Read the model definition and answer for the solid it produces. Units are mm, in the model's axes. Round coordinates to 2 decimals unless told otherwise and drop trailing zeros. Order: outer loops, then holes, each group sorted by start corner. A loop starts at its lowest first (then second) coordinate and runs counter-clockwise, first axis right, second up. Notation, with made-up numbers: M 30.25,73.5 L 40.25,73.5 A18 cw 40.25,94.5 Z; hole C 71,58.5 d10. An arc over 180 degrees is marked long. Use one line per item in the form item = value. Start each with the question number.
Autodesk Inventor part; units mm, degrees
ref_plane "Work Plane1" through (-6.3375, 0, 0) normal (0, -0.8660254, -0.5) x (1, 0, 0)
ref_plane "YZ Plane" through (0, 0, 0) normal (1, 0, 0) x (0, 1, 0)
ref_plane "XZ Plane" through (0, 0, 0) normal (0, 1, 0) x (-1, 0, 0)
sketch "Sketch1" plane through (0, 0, 0) normal (1, 0, 0) x (0, 1, 0)
  line L0 (-3.1754, 0) -> (-1.5877, 2.75)
  line L1 (-1.5877, 2.75) -> (1.5877, 2.75)
  line L2 (1.5877, 2.75) -> (3.1754, 0)
  line L3 (3.1754, 0) -> (1.5877, -2.75)
  line L4 (1.5877, -2.75) -> (-1.5877, -2.75)
  line L5 (-1.5877, -2.75) -> (-3.1754, 0)
  point P0 (0, 0)
  point P1 (0, 0)
  dimension "d0" = 6.3509
extrude "Body" add sketch "Sketch1" along normal blind 2.4
sketch "Sketch2" plane through (0, 0, 0) normal (0, 0, 1) x (1, 0, 0)
  line L0 (0, 1.5877) -> (0, 3.1754)
  line L1 (0, 3.1754) -> (2.4, 3.1754)
  line L2 (2.4, 1.5877) -> (2.4, 3.1754)
  line L3 (-0.16, 0) -> (0.96, 0)
  line L4 (0.1984, 3.1754) -> (0, 2.75)
  line L5 (2.2016, 3.1754) -> (2.4, 2.75)
  dimension "d3" = 25
  dimension "d4" = 25
  dimension "d5" = 5.5
  dimension "d6" = 5.5
revolve "Chamfer1" cut sketch "Sketch2" angle 360 about axis through (-10, 0, 0) along (1, 0, 0)
sketch "Sketch3" plane through (2.4, 0, 0) normal (1, 0, 0) x (0, 0, -1)
  arc A0 (-1.375, -2.3816) -> (1.375, -2.3816) centre (0, 0) ccw
hole "Thread" at (2.4, 0, 0) direction (-1, 0, 0) diameter 1.221 end through all
chamfer "Chamfer2" distance 0.2706 angle 30 1 edges at (2.4, 0, 0.6105) measured on face at (2.4, -2.0253, -0.0245)
chamfer "Chamfer3" distance 0.2706 angle 30 1 edges at (0, 0, 0.6105) measured on face at (0, -2.0253, -0.0245)
ref_plane "Work Plane1" through (-6.3375, 0, 0) normal (0, -0.8660254, -0.5) x (1, 0, 0)
equation "\"d0\" = 1.1547 * SW"
equation "\"d1\" = KOH"
equation "\"d3\" = ANG1"
equation "\"d4\" = ANG2"
equation "\"d5\" = SW0"
equation "\"d6\" = SW01"
equation "\"d8\" = -0.5 * GD1 + 0.5 * NND"
equation "\"d40\" = -0.5 * GD1 + 0.5 * NND"
equation "\"d10\" = -0.5 * GD1 + 0.5 * NND"
equation "\"d41\" = -0.5 * GD1 + 0.5 * NND"
equation "\"ANG1\" = 25deg"
equation "\"ANG2\" = 25deg"
equation "\"NND\" = 3"
equation "\"KOH\" = 2.4"
equation "\"SW\" = 5.5"
equation "\"SW0\" = SW"
equation "\"SW01\" = SW"
equation "\"GUL\" = 0.541266 * PTC"
equation "\"THREADDIA\" = 3"
equation "\"TOA\" = 30deg"
equation "\"PTC\" = 0.5"
equation "\"E0\" = 1.155 * SW"
equation "\"GAL\" = 0.541266 * PTC"
equation "\"SD2\" = 0"
equation "\"WFT\" = 0"
properties part number "ANSI B 18.2.4.1 M - M3 x 0.5" material "Steel, Mild"
Item 1: Find the intervals of material crossed by L1, parallel to Z at x = 1.25, y = 0; L2, parallel to Y at x = 2.1, z = 0.3; L3, parallel to Z at x = 1.55, y = 0.5, in increasing order. Write a range as [from, to].
Item 2: Given P1, Ø1, axis at x = 1.5, z = -1.5, coming from the +Y side; P2, Ø0.7, axis at y = 0, z = 0, coming from the -X side, each flat-ended and moving along its own axis, determine where each tip first touches the part or whether it passes through.
Item 3: Section A-A (x = 2.1) is taken. Write down the section's boundary in (y, z).
Item 4: For a pull along Y with two mould halves and no side action, classify faces 1 (the conical face through (0.07, 1.46, 2.51)), 2 (the conical face through (2.33, -1.46, 2.51)), 3 (the cylindrical face through (1.19, -0.03, 0.61)), 4 (the flat face through (0, -1, 1)) as pulls with the +Y half, pulls with the -Y half, needs draft (parallel to the pull), parting line crosses it, or undercut.
The answers:
q1.L1 = [-2.75, -0.61], [0.61, 2.75]
q1.L2 = [-3, -0.53], [0.53, 3]
q1.L3 = [-2.75, -0.35], [0.35, 2.75]
q2.P1 = 2.6
q2.P2 = through
q3.outline = M -3.18,0 L -1.59,-2.75 L 1.59,-2.75 L 3.18,0 L 1.59,2.75 L -1.59,2.75 Z; hole C 0,0 d1.22
q4.face_1 = pulls with the +Y half
q4.face_2 = pulls with the -Y half
q4.face_3 = undercut
q4.face_4 = needs draft
